Check sheet for the modelled part. Datum: model origin and axes. Units: mm. Round coordinates to 2 decimals unless told otherwise and drop trailing zeros. Order: outer loops, then holes, each group sorted by start corner. A loop starts at its lowest first (then second) coordinate and runs counter-clockwise, first axis right, second up. Notation, with made-up numbers: (42.5, -15) -> (98.5, -15) arc R10 cw to (98.5, -4) -> close; hole circle Ø6 at (10, -29). An arc over 180 degrees is marked (long way). Use CSV: the item, a comma, the result in double quotes.
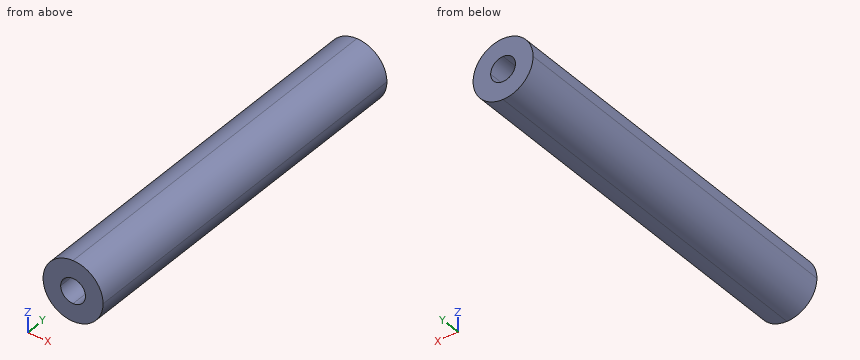
```python
from build123d import *

# Parameters (mm, degrees)
F1_DEPTH = 76.2


with BuildPart() as f1:
    # F0 (on Front) → F1 (new body)
    with BuildSketch(Plane.XZ):
        with BuildLine():
            ThreePointArc((-2.451287, 0), (-1.733322, 1.733322), (0, 2.451287))
            Line((0, 2.451287), (0, 5.930875))
            ThreePointArc((0, 5.930875), (-4.193762, 4.193762), (-5.930875, 0))
            Line((-5.930875, 0), (-2.451287, 0))
        make_face()
        with BuildLine():
            ThreePointArc((0, 2.451287), (1.733322, 1.733322), (2.451287, 0))
            Line((2.451287, 0), (5.930875, 0))
            ThreePointArc((5.930875, 0), (4.193762, 4.193762), (0, 5.930875))
            Line((0, 5.930875), (0, 2.451287))
        make_face()
        with BuildLine():
            Line((0, -5.930875), (0, -2.451287))
            ThreePointArc((0, -2.451287), (-1.733322, -1.733322), (-2.451287, 0))
            Line((-2.451287, 0), (-5.930875, 0))
            ThreePointArc((-5.930875, 0), (-4.193762, -4.193762), (0, -5.930875))
        make_face()
        with BuildLine():
            Line((5.930875, 0), (2.451287, 0))
            ThreePointArc((2.451287, 0), (1.733322, -1.733322), (0, -2.451287))
            Line((0, -2.451287), (0, -5.930875))
            ThreePointArc((0, -5.930875), (4.193762, -4.193762), (5.930875, 0))
        make_face()
    extrude(amount=-F1_DEPTH)


solid = f1.part
```
Q1. Sectioned sample at C-C, the plane x = -1. Enter the section's corners in (y, z), then the cut area to 3 significant figures.
Result sheet:
outline,"(0, -5.85) -> (76.2, -5.85) -> (76.2, -2.24) -> (0, -2.24) -> close; (0, 2.24) -> (76.2, 2.24) -> (76.2, 5.85) -> (0, 5.85) -> close"
area,"550 mm^2"
Q2. Sectioned sample at B-B, the plane z = -1.25. Enter the section's corners in (x, y).
Result sheet:
outline,"(-5.8, 0) -> (-2.11, 0) -> (-2.11, 76.2) -> (-5.8, 76.2) -> close; (2.11, 0) -> (5.8, 0) -> (5.8, 76.2) -> (2.11, 76.2) -> close"
Q3. Sectioned sample at A-A, the plane y = 58. Enter the section's corners in (x, z), then the cut area to 3 significant figures.
Result sheet:
outline,"circle Ø11.86 at (0, 0); hole (-2.45, 0) arc R2.45 ccw to (0, -2.45) arc R2.45 ccw to (2.45, 0) arc R2.45 ccw to (0, 2.45) arc R2.45 ccw to start"
area,"91.6 mm^2"
Q4. Scan lines: L1, parallel to X at y = 38.5, z = 0.25; L2, parallel to Z at x = 1, y = 5; L3, parallel to Z at x = 0.5, y = 59.5. Record each from-to range of solid material in increasing order.
Result sheet:
L1,"x = -5.93 to -2.44, 2.44 to 5.93"
L2,"z = -5.85 to -2.24, 2.24 to 5.85"
L3,"z = -5.91 to -2.4, 2.4 to 5.91"
Q5. Sectioned sample at D-D, the plane x = 3.5. Enter the section's corners in (y, z), then the cut area to 3 significant figures.
Result sheet:
outline,"(0, -4.79) -> (76.2, -4.79) -> (76.2, 4.79) -> (0, 4.79) -> close"
area,"730 mm^2"
Q6. Go/stop test with flat-tipped pins: pin 1 (2 mm diameter, centred on y = 67.5, z = 4.5, fed in from -X); pin 2 (4 mm diameter, centred on x = -3.5, y = 37, fed in from -Z); pin 3 (2 mm diameter, centred on x = 3, y = 32, fed in from -Z). Record where each tip stops, or that it passes through.
Result sheet:
pin 1,"stops at x = -4.79"
pin 2,"stops at z = -5.74"
pin 3,"stops at z = -5.58"
